CAD build for the part. Positions are in the model's coordinates, mm. Give positions to 0.01 mm unless a question says otherwise; leave off trailing zeros. Loops run counter-clockwise (first coordinate to the right, second up) from the corner with the lowest first, then second, coordinate; pieces in that order, holes last. Notation, with made-up numbers: (-7.5, -11.5) - (7.5, -11.5) arc R22 cw to (7.5, 10.5) - close; hole circle Ø2 at (-28.5, 46.5). An arc over 180 degrees is marked (long way). Return JSON: item names as keys, results as strings.
from build123d import *

# Parameters (mm, degrees)
SKETCH1_W             = 110
SKETCH1_H             = 225
BOSS_EXTRUDE1_DEPTH   = 10
M8_CLEARANCE_HOLE1_D  = 8.4
F_8_0MM_DOWEL_HOLE1_D = 8
CUT_EXTRUDE1_REACH    = 127.623
SKETCH8_R             = 7
M6_CLEARANCE_HOLE1_D  = 6.4


with BuildPart() as part:
    # Sketch1 → Boss-Extrude1 (new body)
    with BuildSketch(Plane(origin=(0, 0, 0), x_dir=(1, 0, 0), z_dir=(0, 1, 0))):
        Rectangle(SKETCH1_W, SKETCH1_H)
    extrude(amount=-BOSS_EXTRUDE1_DEPTH)

    # M8 Clearance Hole1 (through all)
    with Locations(Plane(origin=(0, 0, 0), x_dir=(1, 0, 0), z_dir=(0, 1, 0))):
        with Locations((-17, 96.5), (17, 96.5), (-39, -96.5), (39, -96.5)):
            Hole(M8_CLEARANCE_HOLE1_D / 2)

    # Ø8.0mm Dowel Hole1 (through all)
    with Locations(Plane(origin=(0, 0, 0), x_dir=(1, 0, 0), z_dir=(0, 1, 0))):
        with Locations((0, 96.5), (-23.5, -96.5), (23.5, -96.5)):
            Hole(F_8_0MM_DOWEL_HOLE1_D / 2)

    # Sketch8 → Cut-Extrude1 (cut, up to next)
    with BuildSketch(Plane(origin=(0, 0, 0), x_dir=(1, 0, 0), z_dir=(0, 1, 0)), mode=Mode.PRIVATE) as cut_extrude1_sk1:
        with Locations(Location((0, 9.86, 0), (0, 0, 270))):
            Circle(SKETCH8_R)
    cut_extrude1_tool1 = extrude(cut_extrude1_sk1.sketch, amount=-CUT_EXTRUDE1_REACH, mode=Mode.PRIVATE) & part.part
    add(cut_extrude1_tool1.solids().sort_by_distance((0, 0, -9.86))[0], mode=Mode.SUBTRACT)

    # M6 Clearance Hole1 (through all)
    with Locations(Plane(origin=(0, 0, 0), x_dir=(1, 0, 0), z_dir=(0, 1, 0))):
        with Locations((26.75, 23.36), (26.75, -18.64), (-32.25, 42.36), (-32.25, -22.64)):
            Hole(M6_CLEARANCE_HOLE1_D / 2)


solid = part.part
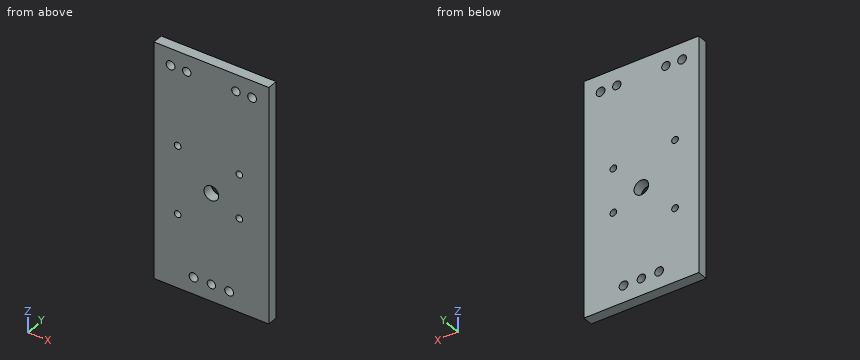
1. Drill centre lines: probe 1 along Z at (x, y) = (-32.25, -7.5); probe 2 along X at (y, z) = (-4, -96.5); probe 3 along X at (y, z) = (-1.75, 96.5). Where is each one in solid material? Low to high.
Values follow:
{"probe 1": "z = -112.5 to -45.56, -39.16 to 19.44, 25.84 to 112.5", "probe 2": "x = -55 to -21.2, -12.8 to -4, 4 to 12.8, 21.2 to 55", "probe 3": "x = -55 to -43.2, -34.8 to -27.5, -19.5 to 19.5, 27.5 to 34.8, 43.2 to 55"}
2. Cut at C-C, the plane x = -17. Write the cut outline in (y, z).
Values follow:
{"outline": "(-10, -112.5) - (0, -112.5) - (0, -100.7) - (-10, -100.7) - close; (-10, -92.3) - (0, -92.3) - (0, 112.5) - (-10, 112.5) - close"}
3. Cut at A-A, the plane z = 96.5. Write the cut outline in (x, y).
Values follow:
{"outline": "(-55, -10) - (-43.2, -10) - (-43.2, 0) - (-55, 0) - close; (-34.8, -10) - (-27.5, -10) - (-27.5, 0) - (-34.8, 0) - close; (-19.5, -10) - (19.5, -10) - (19.5, 0) - (-19.5, 0) - close; (27.5, -10) - (34.8, -10) - (34.8, 0) - (27.5, 0) - close; (43.2, -10) - (55, -10) - (55, 0) - (43.2, 0) - close"}
4. Drop a flat-ended pin along its axis: P1, Ø9.5, axis at x = -17, z = -96.5, coming from the -Y side. Give the stop position or say it passes through.
Values follow:
{"P1": "stops at y = -10"}
5. Cut at D-D, the plane z = -23.36. Write the cut outline in (x, y), plus the area to 3 significant figures.
Values follow:
{"outline": "(-55, -10) - (23.55, -10) - (23.55, 0) - (-55, 0) - close; (29.95, -10) - (55, -10) - (55, 0) - (29.95, 0) - close", "area": "1,040 mm²"}
6. Cut at B-B, the plane y = -4.25. Give the number of separate pieces and of enclosed holes in the cut face, plus the area to 3 significant figures.
Values follow:
{"separate pieces": "1", "enclosed holes": "12", "area": "24,100 mm²"}
